Autodesk Inventor part; units mm, degrees
ref_plane "YZ Plane" through (0, 0, 0) normal (1, 0, 0) x (0, 1, 0)
ref_plane "XZ Plane" through (0, 0, 0) normal (0, 1, 0) x (-1, 0, 0)
ref_plane "XY Plane" through (0, 0, 0) normal (0, 0, 1) x (1, 0, 0)
sketch "Sketch1" plane through (0, 0, 0) normal (0, 0, 1) x (1, 0, 0)
  circle A0 centre (0, 0) radius 8.5725
  dimension "d0" = 17.145
extrude "Extrusion1" add sketch "Sketch1" against normal blind 11.43
sketch "Sketch2" plane through (0, 0, -11.43) normal (0, 0, -1) x (-1, 0, 0)
  circle A0 centre (0, 0) radius 5.5245
  dimension "d3" = 11.049
extrude "Extrusion2" cut sketch "Sketch2" against normal blind 3.81
fillet "Fillet1" radius 1.0583 1 edges at (-8.5725, 0, 0)
ref_plane "Work Plane1" through (0, 0, -8.89) normal (0, 0, -1) x (-1, 0, 0)
sketch "Sketch3" plane through (0, 0, -8.89) normal (0, 0, -1) x (-1, 0, 0)
  circle A0 centre (0, 0) radius 0.635
  dimension "d8" = 1.27
loft "Loft1" add profiles "Sketch3" section 1 edges at (5.5245, 0, -7.62)
sketch "Sketch4" plane through (0, 0, -8.89) normal (0, 0, -1) x (-1, 0, 0)
  circle A0 centre (0, 0) radius 0.635
  circle A1 centre (0, 0) radius 0.9525
  dimension "d13" = 1.905
extrude "Extrusion3" cut sketch "Sketch4" against normal blind 1.27 contours A0
equation "\"d0\" = outsideDiameterForHoleInCat"
equation "\"d1\" = length"
equation "\"d3\" = holeForInteriorButton"
equation "\"d4\" = depthForInteriorButton"
equation "\"d6\" = topFilletRadius"
equation "\"d8\" = offsetCircleDiameter"
equation "\"d13\" = glueHoleDiameter"
equation "\"d14\" = glueHoleDepth"
equation "\"outsideDiameterForHoleInCat\" = 17.145"
equation "\"length\" = 11.43"
equation "\"holeForInteriorButton\" = 11.049"
equation "\"depthForInteriorButton\" = 3.81"
equation "\"planeOffset\" = 0.635"
equation "\"offsetCircleDiameter\" = 1.27"
equation "\"topFilletRadius\" = 1.05833"
equation "\"glueHoleDiameter\" = 1.905"
equation "\"glueHoleDepth\" = 1.27"
properties part number "buttonForCatButton"
Geometry: final body of the model. Coordinates: model frame, mm. A direction names the side the tool comes from. Coordinates: 2 decimals unless noted, no trailing zeros. Order: outer loops, then holes, each group sorted by start corner. A loop starts at its lowest first (then second) coordinate and runs counter-clockwise, first axis right, second up. Notation, with made-up numbers: M 60,76.5 L 82,76.5 A18 ccw 82,91.5 Z; hole C -35,-1.5 d5. An arc over 180 degrees is marked long. Answer as CSV lines item,"result".
Q1. Set-up query: faces 4 (the cylindrical face through (0.08, 0.63, -8.26)), 5 (the flat face through (0, 0, 0)). Return all of +Z, -Z, +X, -X, +Y, -Y with unobstructed straight access to the full face (end or side cutting, diameter ignored); none if empty.
Answers:
face 4,"-Z"
face 5,"+Z, +X, -X, +Y, -Y"
Q2. Draft query along Y for faces 1 (the flat face through (6, 0, -11.43)), 2 (the cylindrical face through (4.609, 7.228, -6.172)), 3 (the conical face through (-0.9, -0.28, -8.81)). Return one class per face: pulls with the +Y half, pulls with the -Y half, needs draft (parallel to the pull), parting line crosses it, or undercut.
Answers:
face 1,"needs draft"
face 2,"parting line crosses it"
face 3,"undercut"
Q3. Section B-B on z = -2. Return the cut outline in (x, y) (1 decimal).
Answers:
outline,"C 0,0 d17.1"
Q4. Section A-A on x = 0. Return the cut outline in (y, z) (1 decimal), and give its area (3 significant figures).
Answers:
outline,"M -8.6,-11.4 L -5.5,-11.4 L -5.5,-7.6 L -0.6,-8.9 L -0.6,-7.6 L 0.6,-7.6 L 0.6,-8.9 L 5.5,-7.6 L 5.5,-11.4 L 8.6,-11.4 L 8.6,-1.1 A1.1 ccw 7.5,0 L -7.5,0 A1.1 ccw -8.6,-1.1 Z"
area,"160 mm^2"
Q5. Line query: probe 1 along X at (y, z) = (2.75, -9.5); probe 2 along Y at (x, z) = (0.75, -11); probe 3 along X at (y, z) = (4.75, -8). Output: solid intervals per line, ascending. Write a range as [from, to].
Answers:
probe 1,"x = [-8.12, -4.79], [4.79, 8.12]"
probe 2,"y = [-8.54, -5.47], [5.47, 8.54]"
probe 3,"x = [-7.14, -2.82], [2.82, 7.14]"
Q6. First-contact query: P1, Ø5, axis at x = -5.5, z = -4, coming from the +Y side; P2, Ø1.5, axis at x = -3.5, z = -1.5, coming from the -Y side; P3, Ø1.4, axis at x = 0, y = 0, coming from the -Z side. Flat tips, straight axial feed; report the tip coordinate or a pass-through.
Answers:
P1,"stops at y = 8.03"
P2,"stops at y = -8.12"
P3,"stops at z = -8.89"
